Source: three-view drawing plus pictorial views. Frame: mm from the lowest corner of the part. A direction names the side the tool comes from. Coordinates: 2 decimals unless noted, no trailing zeros. Loops run counter-clockwise (first coordinate to the right, second up) from the corner with the lowest first, then second, coordinate; pieces in that order, holes last. Notation, with made-up numbers: M 40,88.5 L 89,88.5 A21 cw 89,104.5 Z; hole C 77,76.25 d7. An arc over 180 degrees is marked long. Write each question's results on one line, items separated by ' | '. Start each with the question number.
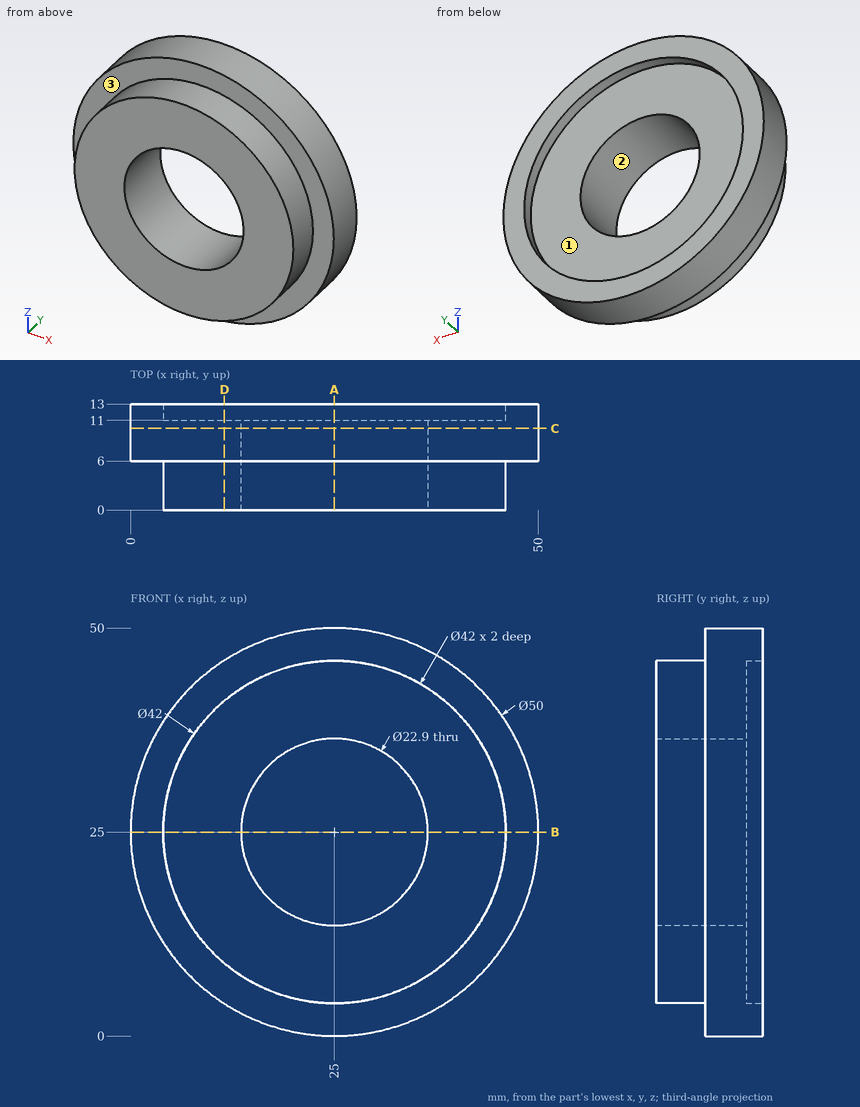
Item 1: Section C-C, the plane y = 10. Return loops of the section in (x, z), plus the area to 3 significant figures.
Item 2: Contact query for flat-ended pins moving along their axis: P1, Ø3, axis at x = 18, y = 10, coming from the +Z side; P2, Ø3, axis at x = 13.5, z = 22.5, coming from the +Y side; P3, Ø6, axis at x = 6, y = 11, coming from the -Z side. Output: stop coordinate, or through.
Item 3: Section B-B, the plane z = 25. Return loops of the section in (x, y).
Item 4: Section A-A, the plane x = 25. Return loops of the section in (y, z).
Item 5: Section D-D, the plane x = 11.5. Return loops of the section in (y, z), plus the area to 3 significant figures.
Item 6: Set-up query: the marked faces 1, 2 and 3. Return all of +Z, -Z, +X, -X, +Y, -Y with unobstructed straight access to the full face (end or side cutting, diameter ignored); none if empty.
Item 7: Ray query, L1, parallel to Z at x = 25, y = 4; L2, parallel to Z at x = 25, y = 11.6; L3, parallel to X at y = 3.25, z = 24. Return the intervals inside material, ascending. Write a range as [from, to].
Solutions:
1) outline: C 25,25 d50; hole C 25,25 d22.9 | area: 1,550 mm²
2) P1: stops at z = 49.39 | P2: stops at y = 11 | P3: stops at z = 5.79
3) outline: M 0,6 L 4,6 L 4,0 L 13.55,0 L 13.55,11 L 4,11 L 4,13 L 0,13 Z; M 36.45,0 L 46,0 L 46,6 L 50,6 L 50,13 L 46,13 L 46,11 L 36.45,11 Z
4) outline: M 0,4 L 6,4 L 6,0 L 13,0 L 13,4 L 11,4 L 11,13.55 L 0,13.55 Z; M 0,36.45 L 11,36.45 L 11,46 L 13,46 L 13,50 L 6,50 L 6,46 L 0,46 Z
5) outline: M 0,8.91 L 6,8.91 L 6,3.96 L 13,3.96 L 13,8.91 L 11,8.91 L 11,41.09 L 13,41.09 L 13,46.04 L 6,46.04 L 6,41.09 L 0,41.09 Z | area: 423 mm²
6) face 1: +Y | face 2: +Y, -Y | face 3: -Y
7) L1: z = [4, 13.55], [36.45, 46] | L2: z = [0, 4], [46, 50] | L3: x = [4.02, 13.59], [36.41, 45.98]
